Geometry check sheet. Reference: the model listing, model coordinates, mm. Face numbers are marked on the shaded views. A direction names the side the tool comes from. Round coordinates to 2 decimals unless told otherwise and drop trailing zeros. Order: outer loops, then holes, each group sorted by start corner. A loop starts at its lowest first (then second) coordinate and runs counter-clockwise, first axis right, second up.
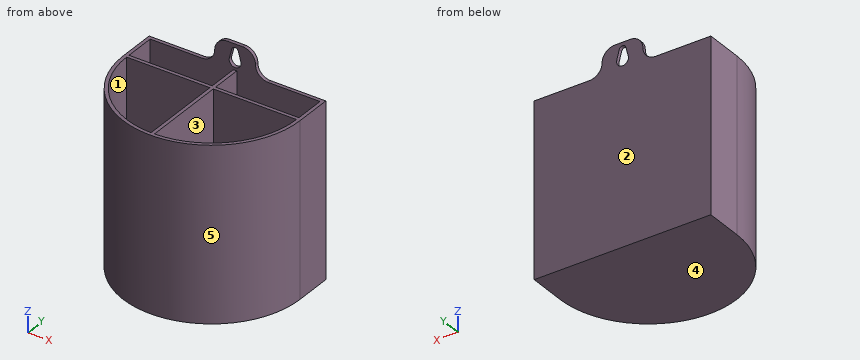
```python
from build123d import *

# Parameters (mm, degrees)
F1_DEPTH = 2
F2_W     = 49
F2_H     = 18
F3_DEPTH = 100
F4_W     = 24
F4_H     = 2
F5_DEPTH = 15
F7_DEPTH = 2
F8_R     = 7.49999


# Not quite as in the source:
# - a fillet or chamfer is up to 0.001 mm smaller than in the source, because OpenCascade refuses the exact size


with BuildPart() as f1:
    # F0 (on Top) → F1 (new body)
    with BuildSketch(Plane.XY):
        with BuildLine():
            Line((104, 0), (0, 0))
            Line((0, 0), (0, -22))
            ThreePointArc((0, -22), (52, -74), (104, -22))
            Line((104, -22), (104, 0))
        make_face()
    extrude(amount=F1_DEPTH)

    # F2 (on face) → F3 (join)
    with BuildSketch(Plane.XY.offset(2)):
        with BuildLine():
            Line((104, 0), (0, 0))
            Line((0, 0), (0, -22))
            ThreePointArc((0, -22), (52, -74), (104, -22))
            Line((104, -22), (104, 0))
        make_face()
        with BuildLine():
            ThreePointArc((51, -71.9899989998), (16.2928578573, -57), (2, -22))
            Line((2, -22), (51, -22))
            Line((51, -22), (51, -71.9899989998))
        make_face(mode=Mode.SUBTRACT)
        with BuildLine():
            ThreePointArc((102, -22), (87.7071421427, -57), (53, -71.9899989998))
            Line((53, -71.9899989998), (53, -22))
            Line((53, -22), (102, -22))
        make_face(mode=Mode.SUBTRACT)
        with Locations((26.5, -11)):
            Rectangle(F2_W, F2_H, mode=Mode.SUBTRACT)
        with Locations((77.5, -11)):
            Rectangle(F2_W, F2_H, mode=Mode.SUBTRACT)
    extrude(amount=F3_DEPTH)

    # F4 (on face) → F5 (join)
    with BuildSketch(Plane.XY.offset(102)):
        with Locations((52, -1)):
            Rectangle(F4_W, F4_H)
    extrude(amount=F5_DEPTH)

    # F6 (on face) → F7 (cut, through all)
    with BuildSketch(Plane.XZ.offset(2)):
        with BuildLine():
            Line((55.3888604279, 107.875), (53.9364916731, 113.5))
            ThreePointArc((53.9364916731, 113.5), (52, 115), (50.0635083269, 113.5))
            Line((50.0635083269, 113.5), (48.6111395721, 107.875))
            ThreePointArc((48.6111395721, 107.875), (52, 103.5), (55.3888604279, 107.875))
        make_face()
    extrude(amount=-F7_DEPTH, mode=Mode.SUBTRACT)

    # F8 (radius 7.5 in the source; OpenCascade refuses exactly that, so slightly less here)
    f8_edges = [f1.edges().sort_by_distance(p)[0] for p in [
        (64, -1, 102),
        (64, -1, 117),
        (40, -1, 102),
        (40, -1, 117),
    ]]
    fillet(f8_edges, radius=F8_R)


solid = f1.part
```
(1) Material ranges on line 1 (X direction, y = -16, z = 16.5); line 2 (Y direction, x = 27, z = 47); line 3 (Y direction, x = 75.5, z = 34.5), recorded low to high.
Returned:
line 1: x = 0 to 2, 51 to 53, 102 to 104
line 2: y = -67.6 to -65.3, -22 to -20, -2 to 0
line 3: y = -68.39 to -66.13, -22 to -20, -2 to 0
(2) Sectioned sample at A-A, the plane z = 90. Record the cut outline in (x, y), and give its area (3 significant figures).
Returned:
outline: (0, -22) arc R52 ccw to (104, -22) - (104, 0) - (0, 0) - close; hole (2, -22) arc R50 ccw to (51, -71.99) - (51, -22) - close; hole (2, -20) - (51, -20) - (51, -2) - (2, -2) - close; hole (53, -71.99) arc R50 ccw to (102, -22) - (53, -22) - close; hole (53, -20) - (102, -20) - (102, -2) - (53, -2) - close
area: 944 mm2
(3) Set-up check for the marked faces 1 and 2: record each of +Z, -Z, +X, -X, +Y, -Y from which the full face is reachable in a straight line by a thin tool's end or side.
Returned:
face 1: +Z
face 2: +Z, -Z, +X, -X, +Y
(4) Sectioned sample at B-B, the plane y = -16. Record the cut outline in (x, z), and give its area (3 significant figures).
Returned:
outline: (0, 0) - (104, 0) - (104, 102) - (102, 102) - (102, 2) - (53, 2) - (53, 102) - (51, 102) - (51, 2) - (2, 2) - (2, 102) - (0, 102) - close
area: 808 mm2
(5) Sectioned sample at C-C, the plane x = 42.5. Record the cut outline in (y, z), and give its area (3 significant figures).
Returned:
outline: (-73.12, 0) - (0, 0) - (0, 115.09) - (-2, 115.09) - (-2, 2) - (-20, 2) - (-20, 102) - (-22, 102) - (-22, 2) - (-71.09, 2) - (-71.09, 102) - (-73.12, 102) - close
area: 776 mm2
(6) Draft check along Y on the marked faces 3, 4 and 5. Enter one of: released by +Y, released by -Y, zero draft, split by the parting line, or undercut.
Returned:
face 3: undercut
face 4: zero draft
face 5: released by -Y
(7) Depth check by flat-ended pin: P1, Ø4, axis at y = -57, z = 69, coming from the -X side; P2, Ø6, axis at y = -35, z = 43.5, coming from the -X side; P3, Ø24.5, axis at x = 14.5, z = 70, coming from the -Y side. Enter the tip coordinate at first touch or a pass-through.
Returned:
P1: stops at x = 11.81
P2: stops at x = 0.97
P3: stops at y = -67.46
